The model under review builds one solid part; all positions refer to its coordinate system, in mm. Face numbers are marked on the shaded views. A direction names the side the tool comes from. Give positions to 0.01 mm unless a question says otherwise; leave off trailing zeros. Order: outer loops, then holes, each group sorted by start corner. A loop starts at its lowest first (then second) coordinate and runs counter-clockwise, first axis right, second up. Notation, with made-up numbers: (81, -11) - (88, -11) arc R19 cw to (88, 11) - close; hole circle Ø5 at (44.5, 66.5). An arc over 180 degrees is marked (long way). Use CSV: the item, a comma, the result in double quotes. Start each with the question number.
1. Machinability: for the marked faces 1, 2, 3 and 4, which of the approach directions +Z, -Z, +X, -X, +Y, -Y give a long, thin tool a straight path to every point of the face, cutting with its end or side? Answer none if there is none.
2. Take a section at A-A, the plane z = 21.5. State the section outline as (x, y) points, then the cut area to 3 significant figures.
3. To check wall thickness, follow line 1 (Y direction, x = -4.95, z = 68.3); line 2 (X direction, y = 8, z = 36); line 3 (Y direction, x = -2.5, z = 60). State the ranges of each line that lie inside material, in increasing order. Write a range as [from, to].
4. Take a section at C-C, the plane y = -0.5. State the section outline as (x, z) points.
5. Draft analysis for pull direction Y (two halves, no side actions). For the marked faces 5, 6 and 7, state which applies: released by +Y, released by -Y, zero draft, split by the parting line, or undercut.
6. Take a section at D-D, the plane x = -4.95. Count the separate pieces of the cut face and the enclosed holes in it, then the cut area to 3 significant figures.
7. For pin 1 (12 mm diameter, centred on x = -5.5, y = 20, fed in from -Z); pin 2 (4 mm diameter, centred on x = -3.5, z = 37, fed in from -Y); pin 3 (1.8 mm diameter, centred on x = 4.95, y = -24.31, fed in from +Z); pin 4 (3.5 mm diameter, centred on x = 1.5, y = -25, fed in from -Z), all flat-tipped, find the tip position at first contact; note any pin that passes through.
8. Take a section at B-B, the plane x = -1.75. State the section outline as (y, z) points, then the cut area to 3 significant figures.
```python
from build123d import *

# Parameters (mm, degrees)
SKETCH_1_W          = 24
SKETCH_1_H          = 24
EXTRUDE_1_DEPTH     = 30
SKETCH_2_W          = 21
SKETCH_2_H          = 21
CUT_EXTRUDE_1_DEPTH = 35.467375879
SKETCH_3_W          = 5
SKETCH_3_H          = 24
EXTRUDE_3_DEPTH     = 2
SKETCH_4_W          = 19
SKETCH_4_H          = 5
EXTRUDE_4_DEPTH     = 2
SKETCH_5_W          = 5
SKETCH_5_H          = 19
EXTRUDE_5_DEPTH     = 2
SKETCH_6_W          = 14
SKETCH_6_H          = 5
EXTRUDE_6_DEPTH     = 2
SKETCH_7_W          = 24
SKETCH_7_H          = 43
EXTRUDE_7_DEPTH     = 28
SKETCH_9_W          = 20
SKETCH_9_H          = 41
CUT_EXTRUDE_2_DEPTH = 27
SKETCH_11_W         = 24
SKETCH_11_H         = 54.3
EXTRUDE_20_DEPTH    = 10
SKETCH_12_W         = 20
SKETCH_12_H         = 41
CUT_EXTRUDE_4_DEPTH = 10
SKETCH_13_R         = 1.5
CUT_EXTRUDE_5_DEPTH = 10
FILLET_2_R          = 5
FILLET_3_R          = 2
CUT_EXTRUDE_START   = -5
CUT_EXTRUDE_6_DEPTH = 5
CUT_EXTRUDE_7_DEPTH = 5
FILLET_4_R          = 1
SKETCH_17_W         = 13.5
SKETCH_17_H         = 24.100930422
CUT_EXTRUDE_8_DEPTH = 45
FILLET_6_R          = 5
EXTRUDE_START       = -1.5
EXTRUDE_23_DEPTH    = 1.5


with BuildPart() as part:
    # 草图1 → 凸台-拉伸1 (new body)
    with BuildSketch(Plane.XY):
        Rectangle(SKETCH_1_W, SKETCH_1_H)
    extrude(amount=EXTRUDE_1_DEPTH)

    # 草图2 → 切除-拉伸1 (cut, through all)
    with BuildSketch(Plane(origin=(0, 0, 0), x_dir=(-1, 0, 0), z_dir=(0, 0, -1))):
        Rectangle(SKETCH_2_W, SKETCH_2_H)
    extrude(amount=-CUT_EXTRUDE_1_DEPTH, mode=Mode.SUBTRACT)

    # 草图3 → 凸台-拉伸3 (add)
    with BuildSketch(Plane.XY.offset(30)):
        with Locations((-9.5, 0)):
            Rectangle(SKETCH_3_W, SKETCH_3_H)
    extrude(amount=EXTRUDE_3_DEPTH)

    # 草图4 → 凸台-拉伸4 (add)
    with BuildSketch(Plane.XY.offset(30)):
        with Locations((2.5, -9.5)):
            Rectangle(SKETCH_4_W, SKETCH_4_H)
    extrude(amount=EXTRUDE_4_DEPTH)

    # 草图5 → 凸台-拉伸5 (add)
    with BuildSketch(Plane.XY.offset(30)):
        with Locations((9.5, 2.5)):
            Rectangle(SKETCH_5_W, SKETCH_5_H)
    extrude(amount=EXTRUDE_5_DEPTH)

    # 草图6 → 凸台-拉伸6 (add)
    with BuildSketch(Plane.XY.offset(30)):
        with Locations((0, 9.5)):
            Rectangle(SKETCH_6_W, SKETCH_6_H)
    extrude(amount=EXTRUDE_6_DEPTH)

    # 草图7 → 凸台-拉伸7 (add)
    with BuildSketch(Plane.XY.offset(32)):
        Rectangle(SKETCH_7_W, SKETCH_7_H)
    extrude(amount=EXTRUDE_7_DEPTH)

    # 草图9 → 切除-拉伸2 (cut)
    with BuildSketch(Plane.XY.offset(60)):
        Rectangle(SKETCH_9_W, SKETCH_9_H)
    extrude(amount=-CUT_EXTRUDE_2_DEPTH, mode=Mode.SUBTRACT)

    # 草图11 → 凸台-拉伸20 (add)
    with BuildSketch(Plane.XY.offset(60)):
        Rectangle(SKETCH_11_W, SKETCH_11_H)
    extrude(amount=EXTRUDE_20_DEPTH)

    # 草图12 → 切除-拉伸4 (cut)
    with BuildSketch(Plane.XY.offset(70)):
        Rectangle(SKETCH_12_W, SKETCH_12_H)
    extrude(amount=-CUT_EXTRUDE_4_DEPTH, mode=Mode.SUBTRACT)

    # 草图13 → 切除-拉伸5 (cut)
    with BuildSketch(Plane.XY.offset(70)):
        with Locations((-4.95, -24.310374207)):
            Circle(SKETCH_13_R)
        with Locations((4.95, -24.310374207)):
            Circle(SKETCH_13_R)
        with Locations(Location((4.95, 24.310374207, 0), (0, 0, 180))):
            Circle(SKETCH_13_R)
        with Locations(Location((-4.95, 24.310374207, 0), (0, 0, 180))):
            Circle(SKETCH_13_R)
    extrude(amount=-CUT_EXTRUDE_5_DEPTH, mode=Mode.SUBTRACT)

    # 圆角2
    fillet_2_edges = [part.edges().sort_by_distance(p)[0] for p in [
        (0, -12, 32),
        (0, 12, 32),
    ]]
    fillet(fillet_2_edges, radius=FILLET_2_R)

    # 圆角3
    fillet_3_edges = [part.edges().sort_by_distance(p)[0] for p in [
        (12, -27.15, 65),
        (12, 27.15, 65),
        (-12, 27.15, 65),
        (-12, -27.15, 65),
    ]]
    fillet(fillet_3_edges, radius=FILLET_3_R)

    # 草图15 → 切除-拉伸6 (cut)
    with BuildSketch(Plane(origin=(0, 0, 60), x_dir=(-1, 0, 0), z_dir=(0, 0, -1)).offset(CUT_EXTRUDE_START)):
        with BuildLine():
            Line((-12, -21.5), (-12, -25.15))
            ThreePointArc((-12, -25.15), (-11.414213562, -26.564213562), (-10, -27.15))
            Line((-10, -27.15), (10, -27.15))
            ThreePointArc((10, -27.15), (11.414213562, -26.564213562), (12, -25.15))
            Line((12, -25.15), (12, -21.5))
            Line((12, -21.5), (-12, -21.5))
        make_face()
    extrude(amount=CUT_EXTRUDE_6_DEPTH, mode=Mode.SUBTRACT)

    # 草图16 → 切除-拉伸7 (cut)
    with BuildSketch(Plane(origin=(0, 0, 60), x_dir=(-1, 0, 0), z_dir=(0, 0, -1)).offset(CUT_EXTRUDE_START)):
        with BuildLine():
            Line((12, 21.5), (12, 25.15))
            ThreePointArc((12, 25.15), (11.414213562, 26.564213562), (10, 27.15))
            Line((10, 27.15), (-10, 27.15))
            ThreePointArc((-10, 27.15), (-11.414213562, 26.564213562), (-12, 25.15))
            Line((-12, 25.15), (-12, 21.5))
            Line((-12, 21.5), (12, 21.5))
        make_face()
    extrude(amount=CUT_EXTRUDE_7_DEPTH, mode=Mode.SUBTRACT)

    # 圆角4
    fillet_4_edges = [part.edges().sort_by_distance(p)[0] for p in [
        (0, -21.5, 65),
        (0, 21.5, 65),
    ]]
    fillet(fillet_4_edges, radius=FILLET_4_R)

    # 草图17 → 切除-拉伸8 (cut)
    with BuildSketch(Plane.ZY.offset(12)):
        with Locations((6.75, 0.050465211)):
            Rectangle(SKETCH_17_W, SKETCH_17_H)
    extrude(amount=-CUT_EXTRUDE_8_DEPTH, mode=Mode.SUBTRACT)

    # 圆角6
    fillet_6_edges = [part.edges().sort_by_distance(p)[0] for p in [
        (12, -12, 20.25),
        (12, 19.25, 32),
        (12, 12, 20.25),
        (12, -13.464466094, 30.535533906),
        (12, 13.464466094, 30.535533906),
        (12, -19.25, 32),
    ]]
    fillet(fillet_6_edges, radius=FILLET_6_R)

    # 草图27 → 凸台-拉伸23 (add)
    with BuildSketch(Plane(origin=(0, 0, 32), x_dir=(-1, 0, 0), z_dir=(0, 0, -1)).offset(EXTRUDE_START)):
        Polygon((-12, 17), (-12, 3.059411708), (-12, -3.059411708), (-12, -17), (-12, -21.5), (12, -21.5), (12, 21.5), (-12, 21.5), align=None)
    extrude(amount=EXTRUDE_23_DEPTH)


solid = part.part
```
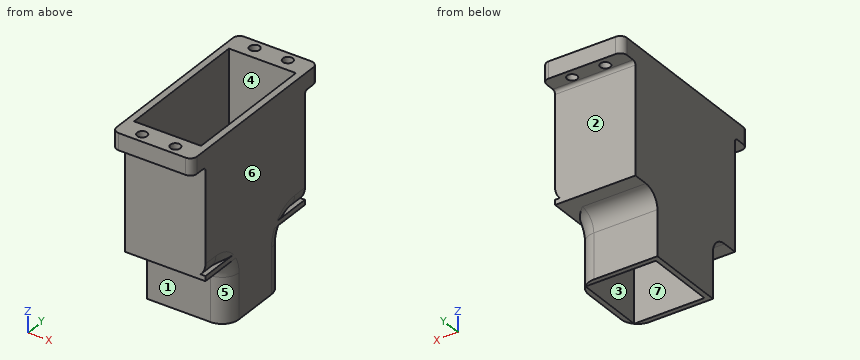
Determined:
1,face 1,"-Z, +X, -X, -Y"
1,face 2,"-Z, +X, -X, +Y"
1,face 3,"-Z"
1,face 4,"+Z"
2,outline,"(-12, -12) - (7, -12) arc R5 ccw to (12, -7) - (12, 7) arc R5 ccw to (7, 12) - (-12, 12) - close; hole (-10.5, -10.5) - (10.5, -10.5) - (10.5, 10.5) - (-10.5, 10.5) - close"
2,area,"124 mm²"
3,line 1,"y = [-27.15, -25.81], [-22.81, -20.5], [20.5, 22.81], [25.81, 27.15]"
3,line 2,"x = [-12, -10], [10, 12]"
3,line 3,"y = [-21.5, -20.5], [20.5, 21.5]"
4,outline,"(-12, 13.5) - (-10.5, 13.5) - (-10.5, 30) - (-7, 30) - (-7, 32) - (7, 32) - (7, 30) - (10.5, 30) - (10.5, 13.5) - (12, 13.5) - (12, 70) - (10, 70) - (10, 33.5) - (-10, 33.5) - (-10, 70) - (-12, 70) - close"
5,face 5,"released by -Y"
5,face 6,"zero draft"
5,face 7,"undercut"
6,separate pieces,"3"
6,enclosed holes,"0"
6,area,"245 mm²"
7,pin 1,"stops at z = 31"
7,pin 2,"stops at y = -21.5"
7,pin 3,"passes through"
7,pin 4,"stops at z = 65"
8,outline,"(-27.15, 65) - (-22.5, 65) arc R1 cw to (-21.5, 64) - (-21.5, 32) - (-17, 32) arc R5 cw to (-12, 27) - (-12, 13.5) - (-10.5, 13.5) - (-10.5, 30) - (-7, 30) - (-7, 32) - (7, 32) - (7, 30) - (10.5, 30) - (10.5, 13.5) - (12, 13.5) - (12, 27) arc R5 cw to (17, 32) - (21.5, 32) - (21.5, 64) arc R1 cw to (22.5, 65) - (27.15, 65) - (27.15, 70) - (20.5, 70) - (20.5, 33.5) - (-20.5, 33.5) - (-20.5, 70) - (-27.15, 70) - close"
8,area,"275 mm²"
